Check sheet for the modelled part. Datum: model origin and axes. Units: mm. Face numbers are marked on the shaded views. A direction names the side the tool comes from. Coordinates: 2 decimals unless noted, no trailing zeros. Order: outer loops, then holes, each group sorted by start corner. A loop starts at its lowest first (then second) coordinate and runs counter-clockwise, first axis right, second up. Notation, with made-up numbers: M 14,63.5 L 58,63.5 A23 ccw 58,77.5 Z; hole C -32.75,-7.5 d1. An arc over 180 degrees is marked long. Answer in a Markdown table with one row per item. Add a question column.
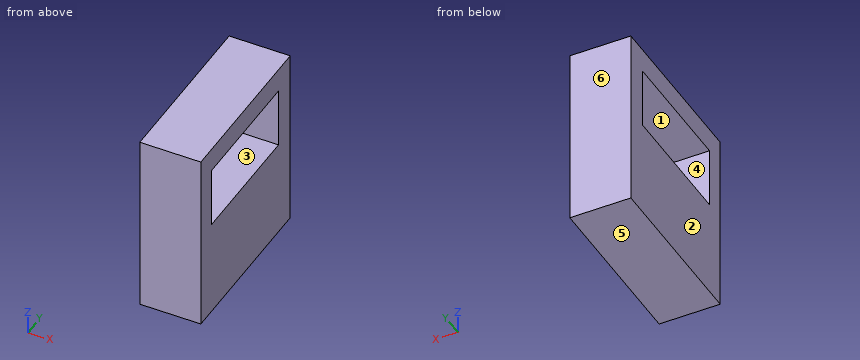
from build123d import *

# Parameters (mm, degrees)
CROQUIS1_W              = 12.7
CROQUIS1_H              = 35.56
SALIENTE_EXTRUIR1_DEPTH = 38.1
CROQUIS3_W              = 12.7
CROQUIS3_H              = 26.67
CORTAR_EXTRUIR1_DEPTH   = 38.1


with BuildPart() as part:
    # Croquis1 → Saliente-Extruir1 (new body)
    with BuildSketch(Plane.XY):
        with Locations((-37.495945778, 19.33754717)):
            Rectangle(CROQUIS1_W, CROQUIS1_H)
    extrude(amount=SALIENTE_EXTRUIR1_DEPTH)

    # Croquis3 → Cortar-Extruir1 (cut)
    with BuildSketch(Plane.ZY.offset(43.845945778)):
        with Locations((26.763723238, 19.135311011)):
            Rectangle(CROQUIS3_W, CROQUIS3_H)
    extrude(amount=-CORTAR_EXTRUIR1_DEPTH, mode=Mode.SUBTRACT)


solid = part.part
1. Section check A-A on x = -39. Enter the section's corners in (y, z).
2. Scan lines: line 1 (Z direction, x = -39.5, y = 18.5); line 2 (Y direction, x = -34.5, z = 31.5). Record each from-to range of solid material in increasing order.
3. Go/stop test with a flat-tipped pin: pin 1 Ø5 at (x, y) = (-34.5, 30.5) entering from -Z. Record where the tip stops, or that it passes through.
4. Section check C-C on z = 32.5. Enter the section's corners in (x, y).
5. Release check for a two-part mould opening along Z. For the marked faces 3, 4, 5 and 6 record: released by +Z, released by -Z, zero draft, split by the parting line, or undercut.
6. Section check B-B on y = 16.5. Enter the section's corners in (x, z), then the cut area to 3 significant figures.
7. Set-up check for the marked faces 1 and 2: record each of +Z, -Z, +X, -X, +Y, -Y from which the full face is reachable in a straight line by a thin tool's end or side.
Result sheet:
| question | item | result |
|---|---|---|
| 1 | outline | M 1.56,0 L 37.12,0 L 37.12,38.1 L 1.56,38.1 Z; hole M 5.8,20.41 L 32.47,20.41 L 32.47,33.11 L 5.8,33.11 Z |
| 2 | line 1 | 0 to 20.41, 33.11 to 38.1 |
| 2 | line 2 | 1.56 to 5.8, 32.47 to 37.12 |
| 3 | pin 1 | z = 0 |
| 4 | outline | M -43.85,1.56 L -31.15,1.56 L -31.15,5.8 L -43.85,5.8 Z; M -43.85,32.47 L -31.15,32.47 L -31.15,37.12 L -43.85,37.12 Z |
| 5 | face 3 | undercut |
| 5 | face 4 | undercut |
| 5 | face 5 | released by -Z |
| 5 | face 6 | zero draft |
| 6 | outline | M -43.85,0 L -31.15,0 L -31.15,20.41 L -43.85,20.41 Z; M -43.85,33.11 L -31.15,33.11 L -31.15,38.1 L -43.85,38.1 Z |
| 6 | area | 323 mm^2 |
| 7 | face 1 | +X, -X |
| 7 | face 2 | +Z, -Z, -X, +Y, -Y |
